from build123d import *

# Parameters (mm, degrees)
ESQUISSE1_W             = 45
ESQUISSE1_H             = 60
BOSS_EXTRU_1_DEPTH      = 27
D_GAGEMENT_M31_D        = 3.2
ESQUISSE4_W             = 30
ESQUISSE4_H             = 10
ENL_V_MAT_EXTRU_1_DEPTH = 27


with BuildPart() as part:
    # Esquisse1 → Boss.-Extru.1 (new body)
    with BuildSketch(Plane(origin=(0, 0, 0), x_dir=(1, 0, 0), z_dir=(0, 1, 0))):
        Rectangle(ESQUISSE1_W, ESQUISSE1_H)
    extrude(amount=BOSS_EXTRU_1_DEPTH)

    # Dégagement M31 (through all)
    with Locations(Plane(origin=(0, 27, 0), x_dir=(1, 0, 0), z_dir=(0, 1, 0))):
        with Locations((-19.05, 25.4), (19.05, 25.4), (19.05, -25.4), (-19.05, -25.4)):
            Hole(D_GAGEMENT_M31_D / 2)

    # Esquisse4 → Enlèv. mat.-Extru.1 (cut)
    with BuildSketch(Plane.XZ):
        with Locations((0, 25)):
            Rectangle(ESQUISSE4_W, ESQUISSE4_H)
    extrude(amount=-ENL_V_MAT_EXTRU_1_DEPTH, mode=Mode.SUBTRACT)


solid = part.part
Model file for the job. Use its own axes, mm. A direction names the side the tool comes from. Round coordinates to 2 decimals unless told otherwise and drop trailing zeros. Loops run counter-clockwise (first coordinate to the right, second up) from the corner with the lowest first, then second, coordinate; pieces in that order, holes last. Notation, with made-up numbers: (41.5, -17.5) - (98.5, -17.5) arc R22 ccw to (98.5, 8.5) - close; hole circle Ø6 at (-14, -16.5). An arc over 180 degrees is marked (long way). Write each question's results on one line, items separated by ' | '.
(1) 3-axis set-ups, long thin cutter, end or side, ignore diameter. For faces 1 (the flat face through (-19, 13, 30)), 2 (the flat face through (-15, 13, 25)): which of +Z, -Z, +X, -X, +Y, -Y reach the whole face in a straight line?
Answer below:
face 1: +Z, +X, -X, +Y, -Y | face 2: +Z, +Y, -Y
(2) Mould opens along Z. For faces 3 (the flat face through (0, 13, -30)), 4 (the flat face through (15, 13, 25)), 5 (the cylindrical face through (-17.8, 13.3, -24.4)) say: released by +Z, released by -Z, zero draft, split by the parting line, or undercut.
Answer below:
face 3: released by -Z | face 4: zero draft | face 5: undercut
(3) Wall check: L1, parallel to Z at x = -19.05, y = 7.25; L2, parallel to X at y = 6.25, z = 25.4; L3, parallel to X at y = 18.75, z = -25.4. Give the ranges that are in metal, low to high.
Answer below:
L1: z = -30 to -27, -23.8 to 23.8, 27 to 30 | L2: x = -22.5 to -20.65, -17.45 to -15, 15 to 17.45, 20.65 to 22.5 | L3: x = -22.5 to -20.65, -17.45 to 17.45, 20.65 to 22.5
(4) Saw through at B-B, the plane x = -19.05. List the corners of the cut face in (y, z), then the cut area to 3 significant figures.
Answer below:
outline: (0, -30) - (27, -30) - (27, -27) - (0, -27) - close; (0, -23.8) - (27, -23.8) - (27, 23.8) - (0, 23.8) - close; (0, 27) - (27, 27) - (27, 30) - (0, 30) - close | area: 1,450 mm^2
(5) Saw through at D-D, the plane z = -25.4. List the corners of the cut face in (x, y), then the cut area to 3 significant figures.
Answer below:
outline: (-22.5, 0) - (-20.65, 0) - (-20.65, 27) - (-22.5, 27) - close; (-17.45, 0) - (17.45, 0) - (17.45, 27) - (-17.45, 27) - close; (20.65, 0) - (22.5, 0) - (22.5, 27) - (20.65, 27) - close | area: 1,040 mm^2
(6) Pin check, flat tips, straight feed: pin 1 (8 mm diameter, centred on x = -12, y = 24, fed in from +Z); pin 2 (1 mm diameter, centred on x = 12.5, y = 17.5, fed in from +Z). Stop position of each tip, or through.
Answer below:
pin 1: stops at z = 30 | pin 2: stops at z = 20
(7) Saw through at A-A, the plane z = 25.4. List the corners of the cut face in (x, y).
Answer below:
outline: (-22.5, 0) - (-20.65, 0) - (-20.65, 27) - (-22.5, 27) - close; (-17.45, 0) - (-15, 0) - (-15, 27) - (-17.45, 27) - close; (15, 0) - (17.45, 0) - (17.45, 27) - (15, 27) - close; (20.65, 0) - (22.5, 0) - (22.5, 27) - (20.65, 27) - close
(8) Saw through at C-C, the plane y = 20.5. List the corners of the cut face in (x, z), then the cut area to 3 significant figures.
Answer below:
outline: (-22.5, -30) - (22.5, -30) - (22.5, 30) - (15, 30) - (15, 20) - (-15, 20) - (-15, 30) - (-22.5, 30) - close; hole circle Ø3.2 at (-19.05, -25.4); hole circle Ø3.2 at (-19.05, 25.4); hole circle Ø3.2 at (19.05, -25.4); hole circle Ø3.2 at (19.05, 25.4) | area: 2,370 mm^2
